Check sheet for the modelled part. Datum: model origin and axes. Units: mm. A direction names the side the tool comes from. Round coordinates to 2 decimals unless told otherwise and drop trailing zeros. Order: outer loops, then holes, each group sorted by start corner. A loop starts at its lowest first (then second) coordinate and runs counter-clockwise, first axis right, second up. Notation, with made-up numbers: (40, 89.25) -> (85, 89.25) arc R23 cw to (85, 98.25) -> close; hole circle Ø5 at (-33, 5.5). An arc over 180 degrees is marked (long way). Use CSV: the item, a comma, the result in double quotes.
```python
from build123d import *

# Parameters (mm, degrees)
SKETCH1_W           = 58
SKETCH1_H           = 74.913224731
SKETCH1_R           = 5
SKETCH1_R_2         = 0.975
SKETCH1_R_3         = 3.2
BOSS_EXTRUDE1_DEPTH = 3
SKETCH6_W           = 58
SKETCH6_H           = 74.913224731
SKETCH6_R           = 1.5
BOSS_EXTRUDE5_DEPTH = 15.2
SKETCH7_R           = 8
SKETCH7_R_2         = 5
BOSS_EXTRUDE6_DEPTH = 4
SKETCH2_R           = 1.5
CUT_EXTRUDE7_DEPTH  = 7
SKETCH5_R           = 2
CUT_EXTRUDE8_DEPTH  = 7
FILLET1_R           = 5
BOSS_EXTRUDE7_START = -5.01
SKETCH8_R           = 4
SKETCH8_R_2         = 0.975
BOSS_EXTRUDE7_DEPTH = 5.01


with BuildPart() as part:
    # Sketch1 → Boss-Extrude1 (new body)
    with BuildSketch(Plane(origin=(0, 0, 0), x_dir=(1, 0, 0), z_dir=(0, 1, 0))):
        with Locations((0, -16.456612366)):
            Rectangle(SKETCH1_W, SKETCH1_H)
        with Locations(Location((0, 0, 0), (0, 0, 270))):
            Circle(SKETCH1_R, mode=Mode.SUBTRACT)
        with Locations(Location((10, -13.747727085, 0), (0, 0, 270))):
            Circle(SKETCH1_R_2, mode=Mode.SUBTRACT)
        with Locations(Location((-3.304338666, -24.330475908, 0), (0, 0, 270))):
            Circle(SKETCH1_R_2, mode=Mode.SUBTRACT)
        with Locations(Location((10, -34.913224731, 0), (0, 0, 270))):
            Circle(SKETCH1_R_3, mode=Mode.SUBTRACT)
    extrude(amount=BOSS_EXTRUDE1_DEPTH)

    # Sketch6 → Boss-Extrude5 (add)
    with BuildSketch(Plane(origin=(0, 0, 0), x_dir=(1, 0, 0), z_dir=(0, 1, 0))):
        with Locations((0, -16.456612366)):
            Rectangle(SKETCH6_W, SKETCH6_H)
        with Locations(Location((24.71466455, 15.465029351, 0), (0, 0, 270))):
            Circle(SKETCH6_R, mode=Mode.SUBTRACT)
        with Locations(Location((24.71466455, -48.378254082, 0), (0, 0, 270))):
            Circle(SKETCH6_R, mode=Mode.SUBTRACT)
        with Locations(Location((-24.71466455, 15.465029351, 0), (0, 0, 270))):
            Circle(SKETCH6_R, mode=Mode.SUBTRACT)
        with Locations(Location((-24.71466455, -48.378254082, 0), (0, 0, 270))):
            Circle(SKETCH6_R, mode=Mode.SUBTRACT)
        with BuildLine():
            Line((-19.24074398, -48.913224731), (19.24074398, -48.913224731))
            ThreePointArc((19.24074398, -48.913224731), (20.408888756, -44.956223279), (24, -42.924883145))
            Line((24, -42.924883145), (24, 10.011658414))
            ThreePointArc((24, 10.011658414), (20.408888756, 12.042998549), (19.24074398, 16))
            Line((19.24074398, 16), (-19.24074398, 16))
            ThreePointArc((-19.24074398, 16), (-20.408888756, 12.042998549), (-24, 10.011658414))
            Line((-24, 10.011658414), (-24, -42.924883145))
            ThreePointArc((-24, -42.924883145), (-20.408888756, -44.956223279), (-19.24074398, -48.913224731))
        make_face(mode=Mode.SUBTRACT)
    extrude(amount=-BOSS_EXTRUDE5_DEPTH)

    # Sketch7 → Boss-Extrude6 (add)
    with BuildSketch(Plane.XZ):
        with Locations(Location((10, 34.913224731, 0), (0, 0, 90))):
            Circle(SKETCH7_R)
        with Locations(Location((10, 34.913224731, 0), (0, 0, 270))):
            Circle(SKETCH7_R_2, mode=Mode.SUBTRACT)
    extrude(amount=BOSS_EXTRUDE6_DEPTH)

    # Sketch2 → Cut-Extrude7 (cut)
    with BuildSketch(Plane(origin=(0, 0, 0), x_dir=(1, 0, 0), z_dir=(0, 1, 0))):
        with Locations(Location((-10.825317547, -6.25, 0), (0, 0, 270))):
            Circle(SKETCH2_R)
        with Locations(Location((-10.825317547, 6.25, 0), (0, 0, 270))):
            Circle(SKETCH2_R)
        with Locations(Location((0, 12.5, 0), (0, 0, 270))):
            Circle(SKETCH2_R)
        with Locations(Location((10.825317547, 6.25, 0), (0, 0, 270))):
            Circle(SKETCH2_R)
    extrude(amount=CUT_EXTRUDE7_DEPTH, mode=Mode.SUBTRACT)

    # Sketch5 → Cut-Extrude8 (cut)
    with BuildSketch(Plane(origin=(29, 0, 0), x_dir=(0, 0, -1), z_dir=(1, 0, 0))):
        with Locations((-31.913224731, -2.1)):
            Circle(SKETCH5_R)
        with Locations((-31.913224731, -10.1)):
            Circle(SKETCH5_R)
        with Locations((-11.913224731, -10.1)):
            Circle(SKETCH5_R)
        with Locations((-11.913224731, -2.1)):
            Circle(SKETCH5_R)
    cut_extrude8 = extrude(amount=-CUT_EXTRUDE8_DEPTH, mode=Mode.SUBTRACT)

    # Mirror1: Cut-Extrude8 across plane
    add(cut_extrude8.mirror(Plane(origin=(0, 0, 0), x_dir=(0, 0, 1), z_dir=(1, 0, 0))), mode=Mode.SUBTRACT)

    # Fillet1
    fillet1_edges = [part.edges().sort_by_distance(p)[0] for p in [
        (29, -6.1, 53.913224731),
        (-29, -6.1, 53.913224731),
        (-29, -6.1, -21),
        (29, -6.1, -21),
    ]]
    fillet(fillet1_edges, radius=FILLET1_R)

    # Sketch8 → Boss-Extrude7 (add)
    with BuildSketch(Plane(origin=(0, 0, 0), x_dir=(1, 0, 0), z_dir=(0, 1, 0)).offset(BOSS_EXTRUDE7_START)):
        with Locations(Location((-3.304338666, -24.330475908, 0), (0, 0, 270))):
            Circle(SKETCH8_R)
        with Locations(Location((-3.304338666, -24.330475908, 0), (0, 0, 270))):
            Circle(SKETCH8_R_2, mode=Mode.SUBTRACT)
    extrude(amount=BOSS_EXTRUDE7_DEPTH)


solid = part.part
```
Q1. Sectioned sample at A-A, the plane z = -6.25. Enter the section's corners in (x, y), then the cut area to 3 significant figures.
Result sheet:
outline,"(-29, -15.2) -> (-24, -15.2) -> (-24, 0) -> (-12.33, 0) -> (-12.33, 3) -> (-29, 3) -> close; (-9.33, 0) -> (9.33, 0) -> (9.33, 3) -> (-9.33, 3) -> close; (12.33, 0) -> (24, 0) -> (24, -15.2) -> (29, -15.2) -> (29, 3) -> (12.33, 3) -> close"
area,"308 mm^2"
Q2. Sectioned sample at C-C, the plane y = -6.5. Enter the section's corners in (x, z), then the cut area to 3 significant figures.
Result sheet:
outline,"(-29, -16) arc R5 ccw to (-24, -21) -> (24, -21) arc R5 ccw to (29, -16) -> (29, 48.91) arc R5 ccw to (24, 53.91) -> (-24, 53.91) arc R5 ccw to (-29, 48.91) -> close; hole circle Ø3 at (-24.71, -15.47); hole circle Ø3 at (-24.71, 48.38); hole (-24, -10.01) arc R5.5 cw to (-19.24, -16) -> (19.24, -16) arc R5.5 cw to (24, -10.01) -> (24, 42.92) arc R5.5 cw to (19.24, 48.91) -> (-19.24, 48.91) arc R5.5 cw to (-24, 42.92) -> close; hole circle Ø3 at (24.71, -15.47); hole circle Ø3 at (24.71, 48.38)"
area,"1,270 mm^2"
Q3. Sectioned sample at B-B, the plane z = 6.25. Enter the section's corners in (x, y), then the cut area to 3 significant figures.
Result sheet:
outline,"(-29, -15.2) -> (-24, -15.2) -> (-24, 0) -> (-12.33, 0) -> (-12.33, 3) -> (-29, 3) -> close; (-9.33, 0) -> (24, 0) -> (24, -15.2) -> (29, -15.2) -> (29, 3) -> (-9.33, 3) -> close"
area,"317 mm^2"
Q4. Access from +Z, -Z, +X, -X, +Y, -Y to the whole of each face (thin tool, end or side, straight path). Record for faces 5 (the face through (-4.88, 1.48, -1.08)), 6 (the face through (-24, -7, 16)).
Result sheet:
face 5,"+Y, -Y"
face 6,"-Y"
Q5. Go/stop test with flat-tipped pins: pin 1 (0.9 mm diameter, centred on x = -24.5, z = 48, fed in from -Y); pin 2 (6 mm diameter, centred on x = 0, z = 0, fed in from -Y); pin 3 (5 mm diameter, centred on x = 7.5, z = 37.5, fed in from -Y). Record where each tip stops, or that it passes through.
Result sheet:
pin 1,"stops at y = 0"
pin 2,"passes through"
pin 3,"stops at y = -4"
Q6. Sectioned sample at D-D, the plane x = 22. Enter the section's corners in (y, z), then the cut area to 3 significant figures.
Result sheet:
outline,"(-15.2, -21) -> (3, -21) -> (3, 53.91) -> (-15.2, 53.91) -> (-15.2, 43.59) -> (0, 43.59) -> (0, -10.68) -> (-15.2, -10.68) -> close"
area,"538 mm^2"
Q7. Mould release check, pull along Z, two halves, no side actions. Record for faces 1 (the face through (29, -6, 17)), 2 (the face through (26.54, -2.01, 33.91)), 3 (the face through (-26.54, -3.32, 13.5)), 4 (the face through (-27.574, -5.973, 52.41)): pulls with the +Z half, pulls with the -Z half, needs draft (parallel to the pull), parting line crosses it, or undercut.
Result sheet:
face 1,"needs draft"
face 2,"undercut"
face 3,"undercut"
face 4,"pulls with the +Z half"
Q8. Scan lines: L1, parallel to X at y = -1.5, z = 19; L2, parallel to Z at x = -15, y = -6.25; L3, parallel to X at y = 1.35, z = 6.25. Record each from-to range of solid material in increasing order.
Result sheet:
L1,"x = -29 to -24, 24 to 29"
L2,"z = -21 to -16, 48.91 to 53.91"
L3,"x = -29 to -12.33, -9.33 to 29"
